Source: CAD feature listing. Evaluate the final solid. Frame: model axes, mm. A direction names the side the tool comes from. Give positions to 0.01 mm unless a question says otherwise; leave off trailing zeros. Write each loop counter-clockwise with the first axis right and the second up, starting at its lowest first coordinate (ties: lowest second). Pieces come first, ordered by that corner, then holes. Notation, with made-up numbers: (-32, 24.25) - (21, 24.25) arc R12 cw to (21, 31.25) - close; hole circle Ø8 at (23, 33.25). An arc over 180 degrees is marked (long way). One line per question, with ' | ' between items. Start each with the question number.
(1) Section B-B, the plane z = 9. Return loops of the section in (x, y).
(2) Pin query (flat end, axial travel): pin 1 (3.5 mm diameter, centred on x = 12, y = -37, fed in from +Z); pin 2 (1 mm diameter, centred on x = 2, z = 4.5, fed in from -Y); pin 3 (2 mm diameter, centred on y = -41, z = 3.5, fed in from -X). Return the tip coordinate at first contact, or that it passes through.
(3) Ray query, line 1 (Z direction, x = -10.5, y = -54.25); line 2 (Y direction, x = 0.5, z = 10.75); line 3 (Y direction, x = 3, z = 12). Return the intervals inside material, ascending. Write a range as [from, to].
(4) Draft query along X for faces 1 (the flat face through (0, -57, 13)), 2 (the flat face through (-15.739, -53, 5)), 3 (the cylindrical face through (11.44, -34.765, 4.479)), 4 (the cylindrical face through (11.1, -37.53, 1.48)). Return one class per face: +X half, -X half, draft (parallel to the pull), parting line (faces both ways), or undercut.
(5) Section A-A, the plane y = -38.5. Return loops of the section in (x, z), plus the area to 3 significant figures.
(6) Access query for faces 5 (the cylindrical face through (0, -56, 9)), 6 (the flat face through (7, -31.046, 3)), 7 (the flat face through (13, -37, 3)). Directions: +Z, -Z, +X, -X, +Y, -Y. A direction counts if a zero-diameter tool reaches every point of the face in a straight line with its end or side. Return the directions, or none.
(7) Section C-C, the plane x = 6.5. Return loops of the section in (y, z), plus the area to 3 significant figures.
(8) Section D-D, the plane z = 5.5. Return loops of the section in (x, y).
```python
from build123d import *

# Parameters (mm, degrees)
F0_R     = 0.8
F1_DEPTH = 3
F2_R     = 2.3
F3_DEPTH = 3
F5_DEPTH = 7
F6_R     = 16
F7_R     = 3


with BuildPart() as f1:
    # F0 (on Top) → F1 (new body)
    with BuildSketch(Plane.XY):
        with BuildLine():
            Line((15.7390861437, -56.8619483254), (15.7390861437, -31.0455008498))
            Line((15.7390861437, -31.0455008498), (-15.7390861437, -31.0455008498))
            Line((-15.7390861437, -31.0455008498), (-15.7390861437, -56.8619483254))
            ThreePointArc((-15.7390861437, -56.8619483254), (0, -59), (15.7390861437, -56.8619483254))
        make_face()
        with Locations((11.7390861437, -37.0455008498)):
            Circle(F0_R, mode=Mode.SUBTRACT)
    extrude(amount=F1_DEPTH)

    # F2 (on face) → F3 (join)
    with BuildSketch(Plane.XY.offset(3)):
        with BuildLine():
            Line((-15.7390861437, -31.0455008498), (-15.7390861437, -56.8619483254))
            ThreePointArc((-15.7390861437, -56.8619483254), (0, -59), (15.7390861437, -56.8619483254))
            Line((15.7390861437, -56.8619483254), (15.7390861437, -31.0455008498))
            Line((15.7390861437, -31.0455008498), (-15.7390861437, -31.0455008498))
        make_face()
        with Locations((11.7390861437, -37.0455008498)):
            Circle(F2_R, mode=Mode.SUBTRACT)
    extrude(amount=F3_DEPTH)

    # F4 (on face) → F5 (join)
    with BuildSketch(Plane.XY.offset(6)):
        with BuildLine():
            ThreePointArc((15.7390861437, -53.7427312979), (0, -56), (-15.7390861437, -53.7427312979))
            Line((-15.7390861437, -53.7427312979), (-15.7390861437, -56.8619483254))
            ThreePointArc((-15.7390861437, -56.8619483254), (0, -59), (15.7390861437, -56.8619483254))
            Line((15.7390861437, -56.8619483254), (15.7390861437, -53.7427312979))
        make_face()
    extrude(amount=F5_DEPTH)

    # F6
    f6_edges = [f1.edges().sort_by_distance(p)[0] for p in [
        (-15.739086, -31.045501, 3),
    ]]
    fillet(f6_edges, radius=F6_R)

    # F7
    f7_edges = [f1.edges().sort_by_distance(p)[0] for p in [
        (15.739086, -31.045501, 3),
    ]]
    fillet(f7_edges, radius=F7_R)


solid = f1.part
```
Check sheet entries:
1) outline: (-15.74, -56.86) arc R59 ccw to (15.74, -56.86) - (15.74, -53.74) arc R56 cw to (-15.74, -53.74) - close
2) pin 1: z = 3 | pin 2: y = -58.98 | pin 3: x = -14.92
3) line 1: [0, 6] | line 2: [-59, -56] | line 3: [-58.92, -55.92]
4) face 1: draft | face 2: -X half | face 3: undercut | face 4: undercut
5) outline: (-13.27, 0) - (15.74, 0) - (15.74, 6) - (13.52, 6) - (13.52, 3) - (9.96, 3) - (9.96, 6) - (-13.27, 6) - close | area: 163 mm²
6) face 5: +Z, +Y | face 6: +Z, -Z, +X, -X, +Y | face 7: +Z
7) outline: (-58.64, 0) - (-31.05, 0) - (-31.05, 6) - (-55.62, 6) - (-55.62, 13) - (-58.64, 13) - close | area: 187 mm²
8) outline: (-15.74, -56.86) arc R59 ccw to (15.74, -56.86) - (15.74, -34.05) arc R3 ccw to (12.74, -31.05) - (0.26, -31.05) arc R16 ccw to (-15.74, -47.05) - close; hole circle Ø4.6 at (11.74, -37.05)
